from build123d import *

# Parameters (mm, degrees)
F1_DEPTH  = 40
F3_DEPTH  = 60
F5_DEPTH  = 40
F7_DEPTH  = 40
F8_W      = 10
F8_H      = 10
F9_DEPTH  = 40
F10_W     = 10
F10_H     = 10
F11_DEPTH = 40


with BuildPart() as f1:
    # F0 (on Front) → F1 (new body)
    with BuildSketch(Plane.XZ):
        Polygon((0, 40), (0, 0), (60, 0), (60, 40), (40, 40), (40, 10), (20, 10), (20, 40), align=None)
    extrude(amount=F1_DEPTH)

    # F2 (on face) → F3 (cut)
    with BuildSketch(Plane.YZ.offset(60)):
        Polygon((-40, 10), (0, 40), (-40, 40), align=None)
    extrude(amount=-F3_DEPTH, mode=Mode.SUBTRACT)

    # F4 (on face) → F5 (cut)
    with BuildSketch(Plane(origin=(0, -19.2, 25.6), x_dir=(1, 0, 0), z_dir=(0, -0.6, 0.8))):
        Polygon((20, -26), (20, 24), (10, -26), align=None)
    extrude(amount=-F5_DEPTH, mode=Mode.SUBTRACT)

    # F6 (on face) → F7 (cut)
    with BuildSketch(Plane(origin=(0, -19.2, 25.6), x_dir=(1, 0, 0), z_dir=(0, -0.6, 0.8))):
        Polygon((50, -26), (40, 24), (40, -26), align=None)
    extrude(amount=-F7_DEPTH, mode=Mode.SUBTRACT)

    # F8 (on face) → F9 (join)
    with BuildSketch(Plane.XZ.offset(40)):
        with Locations((15, 5)):
            Rectangle(F8_W, F8_H)
    extrude(amount=-F9_DEPTH)

    # F10 (on face) → F11 (join)
    with BuildSketch(Plane.XZ.offset(40)):
        with Locations((45, 5)):
            Rectangle(F10_W, F10_H)
    extrude(amount=-F11_DEPTH)


solid = f1.part
The listing builds one solid part. Answer for the finished solid, in the listing's coordinates (mm). A direction names the side the tool comes from. Coordinates: 2 decimals unless noted, no trailing zeros. Order: outer loops, then holes, each group sorted by start corner. A loop starts at its lowest first (then second) coordinate and runs counter-clockwise, first axis right, second up. Notation, with made-up numbers: (89, -33.5) -> (135, -33.5) arc R12 ccw to (135, -24.5) -> close; hole circle Ø7 at (75.25, -16.5). An arc over 180 degrees is marked (long way). Answer in a Markdown table with one row per item. Add a question column.
Item 1: This flat-tipped pin is pushed along its axis until it touches: P1, Ø8, axis at x = 30.5, y = -23, coming from the +Z side. Where does it stop, or does it pass through?
Item 2: Find section A-A (z = 32.5). Write down the section's boundary in (x, y).
Item 3: Which of the six approach directions +Z, -Z, +X, -X, +Y, -Y give full straight-line access (tool end or side, diameter ignored) to faces 4 (the face through (45.07, -16.38, 19.59)), 5 (the face through (8, -20, 25))?
Item 4: Find section B-B (y = -35). Write down the section's boundary in (x, z), then the cut area to 3 significant figures.
Item 5: Find the intervals of material crossed by L1, parallel to Z at x = 39.5, y = -26.5; L2, parallel to X at y = -28, z = 13; L3, parallel to X at y = -20.5, z = 19, in increasing order. Write a range as from..to.
Item 6: Find section D-D (z = 28). Write down the section's boundary in (x, y), then the cut area to 3 significant figures.
Item 7: Find section C-C (x = 13). Write down the section's boundary in (y, z).
Item 8: Determine the mould class of faces 1 (the face through (15.07, -14.22, 17.88)), 2 (the face through (60, -15, 15)), 3 (the face through (30, -20, 0)) for opening direction X: +X half, -X half, draft (parallel to the pull), parting line (faces both ways), or undercut.
Result set:
| question | item | result |
|---|---|---|
| 1 | P1 | stops at z = 10 |
| 2 | outline | (0, -10) -> (17.5, -10) -> (19.1, 0) -> (0, 0) -> close; (40.9, 0) -> (42.5, -10) -> (60, -10) -> (60, 0) -> close |
| 3 | face 4 | -Y |
| 3 | face 5 | +Z, +X, -X, -Y |
| 4 | outline | (0, 0) -> (60, 0) -> (60, 13.75) -> (48.75, 13.75) -> (49.2, 10) -> (10.8, 10) -> (11.25, 13.75) -> (0, 13.75) -> close |
| 4 | area | 683 mm² |
| 5 | L1 | z = 0..10 |
| 5 | L2 | x = 0..12.28, 47.72..60 |
| 5 | L3 | x = 0..14.2, 45.8..60 |
| 6 | outline | (0, -16) -> (16, -16) -> (18.56, 0) -> (0, 0) -> close; (41.44, 0) -> (44, -16) -> (60, -16) -> (60, 0) -> close |
| 6 | area | 553 mm² |
| 7 | outline | (-40, 0) -> (0, 0) -> (0, 40) -> (-28, 19) -> (-21.25, 10) -> (-40, 10) -> close |
| 8 | face 1 | undercut |
| 8 | face 2 | +X half |
| 8 | face 3 | draft |
